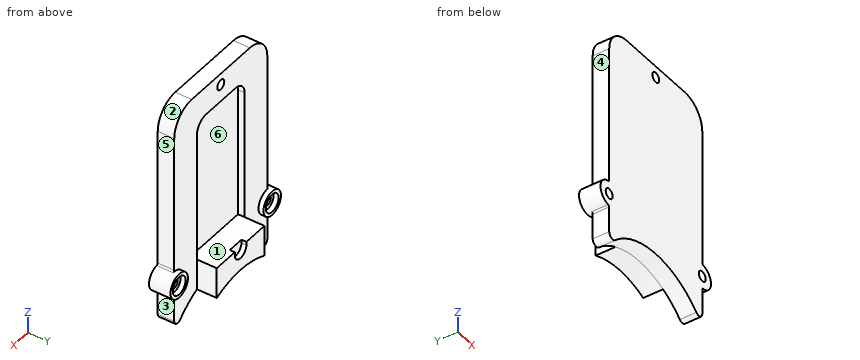
```python
from build123d import *

# Parameters (mm, degrees)
BOSS_EXTRUDE1_DEPTH                     = 10
SKETCH2_R                               = 7.5
BOSS_EXTRUDE2_DEPTH                     = 13
BOSS_EXTRUDE3_DEPTH                     = 12
SKETCH4_W                               = 41
SKETCH4_H                               = 87
CUT_EXTRUDE1_DEPTH                      = 4
CUT_EXTRUDE2_DEPTH                      = 3
CBORE_FOR_M5_HEX_HEAD_BOLT1_D           = 6
CBORE_FOR_M5_HEX_HEAD_BOLT1_CBORE_D     = 11
CBORE_FOR_M5_HEX_HEAD_BOLT1_CBORE_DEPTH = 3
SKETCH8_R                               = 3
CUT_EXTRUDE3_DEPTH                      = 176.958091601
FILLET1_R                               = 8
FILLET2_R                               = 1


with BuildPart() as part:
    # Sketch1 → Boss-Extrude1 (new body)
    with BuildSketch(Plane(origin=(0, 0, 0), x_dir=(1, 0, 0), z_dir=(0, 1, 0))):
        with BuildLine():
            Line((25, -169), (-25, -169))
            ThreePointArc((-25, -169), (-35.606601718, -164.606601718), (-40, -154))
            Line((-40, -154), (-40, -37.947331922))
            ThreePointArc((-40, -37.947331922), (-38.165543035, -35.183003896), (-34.905660377, -35.799369738))
            ThreePointArc((-34.905660377, -35.799369738), (0, -50), (34.905660377, -35.799369738))
            ThreePointArc((34.905660377, -35.799369738), (38.165543035, -35.183003896), (40, -37.947331922))
            Line((40, -37.947331922), (40, -154))
            ThreePointArc((40, -154), (35.606601718, -164.606601718), (25, -169))
        make_face()
    extrude(amount=BOSS_EXTRUDE1_DEPTH)

    # Sketch2 → Boss-Extrude2 (add)
    with BuildSketch(Plane(origin=(0, 0, 0), x_dir=(1, 0, 0), z_dir=(0, 1, 0))):
        with Locations(Location((40, -62, 0), (0, 0, 270))):
            Circle(SKETCH2_R)
    boss_extrude2 = extrude(amount=BOSS_EXTRUDE2_DEPTH)

    # Sketch3 → Boss-Extrude3 (add)
    with BuildSketch(Plane(origin=(0, 10, 0), x_dir=(1, 0, 0), z_dir=(0, 1, 0))):
        with BuildLine():
            Line((-20.5, -45.604276115), (-20.5, -64.5))
            Line((-20.5, -64.5), (20.5, -64.5))
            Line((20.5, -64.5), (20.5, -45.604276115))
            ThreePointArc((20.5, -45.604276115), (0, -50), (-20.5, -45.604276115))
        make_face()
    extrude(amount=BOSS_EXTRUDE3_DEPTH)

    # Sketch4 → Cut-Extrude1 (cut)
    with BuildSketch(Plane(origin=(0, 10, 0), x_dir=(1, 0, 0), z_dir=(0, 1, 0))):
        with Locations((0, -108)):
            Rectangle(SKETCH4_W, SKETCH4_H)
    extrude(amount=-CUT_EXTRUDE1_DEPTH, mode=Mode.SUBTRACT)

    # Sketch5 → Cut-Extrude2 (cut)
    with BuildSketch(Plane(origin=(0, 22, 0), x_dir=(1, 0, 0), z_dir=(0, 1, 0))):
        with BuildLine():
            Line((-5, -64.5), (-5, -62.5))
            ThreePointArc((-5, -62.5), (0, -57.5), (5, -62.5))
            Line((5, -62.5), (5, -64.5))
            Line((5, -64.5), (-5, -64.5))
        make_face()
    extrude(amount=-CUT_EXTRUDE2_DEPTH, mode=Mode.SUBTRACT)

    # CBORE for M5 Hex Head Bolt1 (through all)
    with Locations(Plane(origin=(0, 13, 0), x_dir=(1, 0, 0), z_dir=(0, 1, 0))):
        with Locations((40, -62)):
            cbore_for_m5_hex_head_bolt1 = CounterBoreHole(CBORE_FOR_M5_HEX_HEAD_BOLT1_D / 2, CBORE_FOR_M5_HEX_HEAD_BOLT1_CBORE_D / 2, CBORE_FOR_M5_HEX_HEAD_BOLT1_CBORE_DEPTH)

    # Mirror3: Boss-Extrude2, CBORE for M5 Hex Head Bolt1 across plane
    add(boss_extrude2.mirror(Plane(origin=(0, 0, 0), x_dir=(0, 0, 1), z_dir=(1, 0, 0))))
    add(cbore_for_m5_hex_head_bolt1.mirror(Plane(origin=(0, 0, 0), x_dir=(0, 0, 1), z_dir=(1, 0, 0))), mode=Mode.SUBTRACT)

    # Sketch8 → Cut-Extrude3 (cut, through all)
    with BuildSketch(Plane(origin=(0, 10, 0), x_dir=(1, 0, 0), z_dir=(0, 1, 0))):
        with Locations(Location((0, -162, 0), (0, 0, 270))):
            Circle(SKETCH8_R)
    extrude(amount=-CUT_EXTRUDE3_DEPTH, mode=Mode.SUBTRACT)

    # Fillet1
    fillet1_edges = [part.edges().sort_by_distance(p)[0] for p in [
        (-20.5, 8, 151.5),
        (20.5, 8, 151.5),
    ]]
    fillet(fillet1_edges, radius=FILLET1_R)

    # Fillet2
    # the kernel refuses this fillet: 1 mm, written as the material it adds along each edge
    with BuildSketch(Plane(origin=(40, 10, 54.5), x_dir=(0, 0, -1), z_dir=(0, -1, 0))) as fillet2_piece_1:
        with BuildLine():
            CenterArc((0.940971508, 1), FILLET2_R, 186.756327031, 83.243672969)
            ThreePointArc((-0.052083963, 0.882352941), (-0.013032314, 0.441944412), (0, 0))
            Line((0, 0), (0.940971508, 0))
        make_face()
    extrude(amount=10)
    with BuildSketch(Plane(origin=(40, 0, 69.5), x_dir=(0.9982623581847863, 0, -0.058925921557066524), z_dir=(0, 1, 0))) as fillet2_piece_2:
        with BuildLine():
            CenterArc((0.942814745, -0.998262358), FILLET2_R, 93.378163515, 83.243672969)
            Line((-0.055447613, -0.939336437), (0, 0))
            ThreePointArc((0, 0), (0.441944412, -0.013032314), (0.883888823, 0))
        make_face()
    extrude(amount=10)
    with BuildSketch(Plane(origin=(-40, 10, 54.5), x_dir=(0, 0, -1), z_dir=(0, -1, 0))) as fillet2_piece_3:
        with BuildLine():
            CenterArc((0.940971508, -1), FILLET2_R, 90, 83.243672969)
            ThreePointArc((-0.052083963, -0.882352941), (-0.013032314, -0.441944412), (0, 0))
            Line((0, 0), (0.940971508, 0))
        make_face()
    extrude(amount=10)
    with BuildSketch(Plane(origin=(-40, 0, 69.5), x_dir=(-0.9982623581847863, 0, -0.05892592155706747), z_dir=(0, 1, 0))) as fillet2_piece_4:
        with BuildLine():
            CenterArc((0.942814745, 0.998262358), FILLET2_R, 183.378163515, 83.243672969)
            Line((-0.055447613, 0.939336437), (0, 0))
            ThreePointArc((0, 0), (0.441944412, 0.013032314), (0.883888823, 0))
        make_face()
    extrude(amount=10)


solid = part.part
```
Verification items for the finished model (mm, model axes). Face numbers are marked on the shaded views. A direction names the side the tool comes from. Coordinates: 2 decimals unless noted, no trailing zeros. Order: outer loops, then holes, each group sorted by start corner. A loop starts at its lowest first (then second) coordinate and runs counter-clockwise, first axis right, second up. Notation, with made-up numbers: (-3, -14.5) - (28, -14.5) arc R12 cw to (28, -10.5) - close; hole circle Ø6 at (88, -37). An arc over 180 degrees is marked (long way). Return JSON: item names as keys, results as strings.
(1) Section check C-C, the plane z = 110. Record the cut outline in (x, y).
Filled sheet:
{"outline": "(-40, 0) - (40, 0) - (40, 10) - (20.5, 10) - (20.5, 6) - (-20.5, 6) - (-20.5, 10) - (-40, 10) - close"}
(2) Section check D-D, the plane x = -18.5. Record the cut outline in (y, z), and give its area (3 significant figures).
Filled sheet:
{"outline": "(0, 46.45) - (22, 46.45) - (22, 64.5) - (6, 64.5) - (6, 148.79) - (10, 148.79) - (10, 169) - (0, 169) - close", "area": "1,100 mm^2"}
(3) Thickness scan on line 1 along X through (y, z) = (6.75, 62); line 2 along Z through (x, y) = (40, 11.4); line 3 along X through (y, z) = (11.9, 62). Record the ranges inside material, lowest first.
Filled sheet:
{"line 1": "x = -47.5 to -43, -37 to 37, 43 to 47.5", "line 2": "z = 54.5 to 56.5, 67.5 to 69.5", "line 3": "x = -47.5 to -45.5, -34.5 to -32.5, -20.5 to 20.5, 32.5 to 34.5, 45.5 to 47.5"}
(4) Go/stop test with flat-tipped pins: pin 1 (6 mm diameter, centred on x = 16.5, y = 5, fed in from -Z); pin 2 (8 mm diameter, centred on x = 8, y = 19.5, fed in from -Z); pin 3 (10 mm diameter, centred on y = 2.5, z = 90.5, fed in from +X); pin 4 (5.5 mm diameter, centred on x = 40, z = 62, fed in from -Y). Record where each tip stops, or that it passes through.
Filled sheet:
{"pin 1": "stops at z = 46.04", "pin 2": "stops at z = 48.54", "pin 3": "stops at x = 40", "pin 4": "passes through"}
(5) Section check B-B, the plane z = 162. Record the cut outline in (x, y), and give its area (3 significant figures).
Filled sheet:
{"outline": "(-37.69, 0) - (-3, 0) - (-3, 10) - (-37.69, 10) - close; (3, 0) - (37.69, 0) - (37.69, 10) - (3, 10) - close", "area": "694 mm^2"}
(6) Mould release check, pull along Z, two halves, no side actions. Record for the marked faces 1, 2 and 3: pulls with the +Z half, pulls with the -Z half, needs draft (parallel to the pull), parting line crosses it, or undercut.
Filled sheet:
{"face 1": "undercut", "face 2": "pulls with the +Z half", "face 3": "needs draft"}
(7) Access from +Z, -Z, +X, -X, +Y, -Y to the whole of each face (thin tool, end or side, straight path). Record for the marked faces 4, 5 and 6.
Filled sheet:
{"face 4": "+Z, -X, +Y, -Y", "face 5": "+Z, +X, +Y, -Y", "face 6": "+Y"}
(8) Section check A-A, the plane y = 3. Record the cut outline in (x, z), and give its area (3 significant figures).
Filled sheet:
{"outline": "(-40.88, 54.55) arc R1 cw to (-40, 53.56) - (-40, 37.95) arc R3 ccw to (-34.91, 35.8) arc R50 cw to (34.91, 35.8) arc R3 ccw to (40, 37.95) - (40, 53.56) arc R1 cw to (40.88, 54.55) arc R7.5 ccw to (40.88, 69.45) arc R1 cw to (40, 70.44) - (40, 154) arc R15 ccw to (25, 169) - (-25, 169) arc R15 ccw to (-40, 154) - (-40, 70.44) arc R1 cw to (-40.88, 69.45) arc R7.5 ccw to start; hole circle Ø6 at (-40, 62); hole circle Ø6 at (0, 162); hole circle Ø6 at (40, 62)", "area": "9,970 mm^2"}
